Read the model definition and answer for the solid it produces. Units are mm, in the model's axes. A direction names the side the tool comes from. Coordinates: 2 decimals unless noted, no trailing zeros. Write each loop counter-clockwise with the first axis right and the second up, starting at its lowest first coordinate (ties: lowest second). Pieces come first, ordered by that corner, then holes.
from build123d import *

# Parameters (mm, degrees)
SKETCH1_R           = 26.67
BOSS_EXTRUDE1_DEPTH = 20.828
SKETCH4_R           = 1.5
SKETCH4_R_2         = 4
CUT_EXTRUDE2_DEPTH  = 21.828
CUT_EXTRUDE3_START  = -10.414
SKETCH5_R           = 26.67
CUT_EXTRUDE3_DEPTH  = 8.509
BOSS_EXTRUDE2_START = 10.414
SKETCH9_R           = 1.5
BOSS_EXTRUDE2_DEPTH = 35


with BuildPart() as part:
    # Sketch1 → Boss-Extrude1 (new body)
    with BuildSketch(Plane.XY):
        Circle(SKETCH1_R)
    extrude(amount=BOSS_EXTRUDE1_DEPTH)

    # Sketch4 → Cut-Extrude2 (cut, through all)
    with BuildSketch(Plane(origin=(0, 0, 0), x_dir=(-1, 0, 0), z_dir=(0, 0, -1))):
        with Locations((0, 10.517)):
            Circle(SKETCH4_R)
        with Locations((9.107989172, -5.2585)):
            Circle(SKETCH4_R)
        with Locations((-9.107989172, -5.2585)):
            Circle(SKETCH4_R)
        Circle(SKETCH4_R_2)
        with BuildLine():
            Line((-3.962833887, 15.486170365), (-15.392833887, -4.311170365))
            ThreePointArc((-15.392833887, -4.311170365), (-16.285992128, -4.744214498), (-17.018969403, -4.074884104))
            ThreePointArc((-17.018969403, -4.074884104), (-15.155444566, 8.75), (-4.98053155, 16.776301901))
            ThreePointArc((-4.98053155, 16.776301901), (-4.034385787, 16.476190157), (-3.962833887, 15.486170365))
        make_face()
        with BuildLine():
            Line((15.392833887, -4.311170365), (3.962833887, 15.486170365))
            ThreePointArc((3.962833887, 15.486170365), (4.034385787, 16.476190157), (4.98053155, 16.776301901))
            ThreePointArc((4.98053155, 16.776301901), (15.155444566, 8.75), (17.018969403, -4.074884104))
            ThreePointArc((17.018969403, -4.074884104), (16.285992128, -4.744214498), (15.392833887, -4.311170365))
        make_face()
        with BuildLine():
            Line((-11.43, -11.175), (11.43, -11.175))
            ThreePointArc((11.43, -11.175), (12.25160634, -11.731975659), (12.038437853, -12.701417798))
            ThreePointArc((12.038437853, -12.701417798), (0, -17.5), (-12.038437853, -12.701417798))
            ThreePointArc((-12.038437853, -12.701417798), (-12.25160634, -11.731975659), (-11.43, -11.175))
        make_face()
    extrude(amount=-CUT_EXTRUDE2_DEPTH, mode=Mode.SUBTRACT)

    # Sketch5 → Cut-Extrude3 (cut, symmetric)
    with BuildSketch(Plane(origin=(0, 0, 0), x_dir=(-1, 0, 0), z_dir=(0, 0, -1)).offset(CUT_EXTRUDE3_START)):
        Circle(SKETCH5_R)
    extrude(amount=CUT_EXTRUDE3_DEPTH, both=True, mode=Mode.SUBTRACT)

    # Sketch9 → Boss-Extrude2 (add)
    with BuildSketch(Plane.XY.offset(10.414).offset(BOSS_EXTRUDE2_START)):
        with Locations((0, 10.517)):
            Circle(SKETCH9_R)
        with Locations((9.107989172, -5.2585)):
            Circle(SKETCH9_R)
        with Locations((-9.107989172, -5.2585)):
            Circle(SKETCH9_R)
    extrude(amount=-BOSS_EXTRUDE2_DEPTH)


solid = part.part
Item 1: The part is cut by section D-D (y = -23). Give the vertices of the cut face in (x, z) (3 decimals), and give its area (3 significant figures).
Item 2: Determine the mould class of faces 1 (the flat face through (-9.758, 5.449, 19.862)), 2 (the cylindrical face through (12.26, -11.75, 0.94)), 3 (the cylindrical face through (-0.325, 9.053, -6.987)), 4 (the flat face through (0, 11, -14.172)) for opening direction Y: +Y half, -Y half, draft (parallel to the pull), parting line (faces both ways), or undercut.
Item 3: Given pin 1 (0.6 mm diameter, centred on x = -3, z = 1, fed in from -Y); pin 2 (2 mm diameter, centred on y = 17.5, z = 0.5, fed in from +X); pin 3 (8 mm diameter, centred on y = 5.5, z = 13.5, fed in from +X), each flat-ended and moving along its own axis, determine where each tip first touches the part or whether it passes through.
Item 4: The part is cut by section C-C (y = 8). Give the vertices of the cut face in (x, z) (3 decimals), and give its area (3 significant figures).
Item 5: The part is cut by section A-A (x = 0). State how many separate pieces and enclosed holes the cut face has, and give its area (3 significant figures).
Item 6: Find the intervals of material crossed by probe 1 along Y at (x, z) = (0, 20.25) (3 decimals); probe 2 along Z at (x, y) = (-18, -3.5) (3 decimals); probe 3 along Y at (x, z) = (1, -4), in increasing order.
Item 7: For faces 5 (the cylindrical face through (7.918, -6.171, -6.987)), 6 (the cylindrical face through (-15.06, 8.91, 0.94)), 7 (the cylindrical face through (-7.72, -5.83, 10.53)), determine the directions among +Z, -Z, +X, -X, +Y, -Y from which every point of the face is accessible in a straight line to the end or side of a thin tool.
Answer:
1. outline: (-13.501, 0) - (13.501, 0) - (13.501, 1.905) - (-13.501, 1.905) - close; (-13.501, 18.923) - (13.501, 18.923) - (13.501, 20.828) - (-13.501, 20.828) - close
1. area: 103 mm2
2. face 1: undercut
2. face 2: undercut
2. face 3: parting line
2. face 4: draft
3. pin 1: stops at y = -26.53
3. pin 2: stops at x = 20.95
3. pin 3: stops at x = 1.1
4. outline: (-25.442, 0) - (-15.564, 0) - (-15.564, 1.905) - (-25.442, 1.905) - close; (-25.442, 18.923) - (-15.564, 18.923) - (-15.564, 20.828) - (-25.442, 20.828) - close; (-8.285, 0) - (8.285, 0) - (8.285, 1.905) - (-8.285, 1.905) - close; (-8.285, 18.923) - (8.285, 18.923) - (8.285, 20.828) - (-8.285, 20.828) - close; (15.564, 0) - (25.442, 0) - (25.442, 1.905) - (15.564, 1.905) - close; (15.564, 18.923) - (25.442, 18.923) - (25.442, 20.828) - (15.564, 20.828) - close
4. area: 138 mm2
5. separate pieces: 5
5. enclosed holes: 0
5. area: 242 mm2
6. probe 1: y = -26.67 to -17.5, -11.175 to -4, 4 to 26.67
6. probe 2: z = 0 to 1.905, 18.923 to 20.828
6. probe 3: y = 9.4 to 11.64
7. face 5: -Z
7. face 6: +Z, -Z
7. face 7: none
